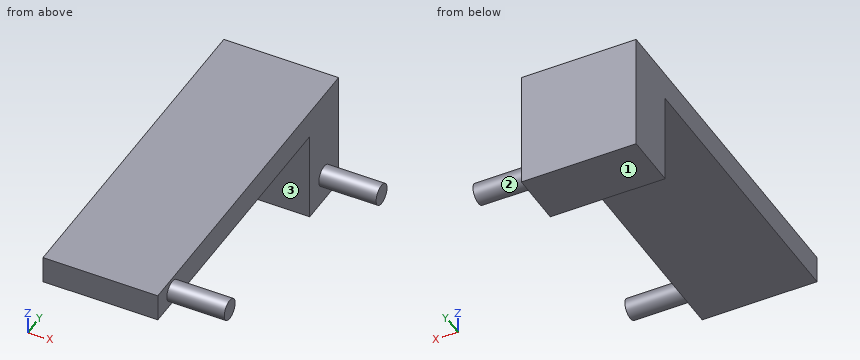
```python
from build123d import *

# Parameters (mm, degrees)
F0_W     = 50
F0_H     = 150
F1_DEPTH = 12
F2_W     = 24
F2_H     = 40
F3_DEPTH = 50
F4_R     = 4.5
F5_DEPTH = 25


with BuildPart() as f1:
    # F0 (on Top) → F1 (new body)
    with BuildSketch(Plane.XY):
        Rectangle(F0_W, F0_H)
    extrude(amount=F1_DEPTH)

    # F2 (on face) → F3 (join)
    with BuildSketch(Plane.YZ.offset(25)):
        with Locations((63, -20)):
            Rectangle(F2_W, F2_H)
    extrude(amount=-F3_DEPTH)

    # F4 (on face) → F5 (join)
    with BuildSketch(Plane.YZ.offset(25)):
        with Locations((-63, 6)):
            Circle(F4_R)
        with Locations((63, -28)):
            Circle(F4_R)
    extrude(amount=F5_DEPTH)


solid = f1.part
```
Check sheet for the modelled part. Datum: model origin and axes. Units: mm. Face numbers are marked on the shaded views. A direction names the side the tool comes from. Give positions to 0.01 mm unless a question says otherwise; leave off trailing zeros. Write each loop counter-clockwise with the first axis right and the second up, starting at its lowest first coordinate (ties: lowest second). Pieces come first, ordered by that corner, then holes. Notation, with made-up numbers: (55.25, -3.75) - (76.25, -3.75) arc R20 ccw to (76.25, 29.25) - close; hole circle Ø6 at (76, 47.5). An arc over 180 degrees is marked (long way). Answer as a JSON object with one key per item and string values. Group by question number.
1) Depth check by flat-ended pin: P1, Ø12, axis at x = -9, z = -25, coming from the -Y side; P2, Ø15, axis at x = 7, y = -32, coming from the -Z side. Enter the tip coordinate at first touch or a pass-through.
2) Sectioned sample at B-B (z = 6). Record the cut outline in (x, y).
3) Thickness scan on probe 1 along Z at (x, y) = (-16, 46); probe 2 along X at (y, z) = (69, -19); probe 3 along Y at (x, z) = (-7, -36). Record the ranges inside material, lowest first. Write a range as from..to.
4) Sectioned sample at A-A (y = 63). Record the cut outline in (x, z), then the cut area to 4 significant figures.
5) Sectioned sample at D-D (y = -16). Record the cut outline in (x, z), then the cut area to 3 significant figures.
6) Access from +Z, -Z, +X, -X, +Y, -Y to the whole of each face (thin tool, end or side, straight path). Record for the marked faces 1, 2 and 3.
7) Sectioned sample at C-C (x = -4.5). Record the cut outline in (y, z).
Geometry results:
{
 "1": {"P1": "stops at y = 51", "P2": "stops at z = 0"},
 "2": {"outline": "(-25, -75) - (25, -75) - (25, -67.5) - (50, -67.5) - (50, -58.5) - (25, -58.5) - (25, 75) - (-25, 75) - close"},
 "3": {"probe 1": "z = 0..12", "probe 2": "x = -25..25", "probe 3": "y = 51..75"},
 "4": {"outline": "(-25, -40) - (25, -40) - (25, -32.5) - (50, -32.5) - (50, -23.5) - (25, -23.5) - (25, 12) - (-25, 12) - close", "area": "2,825 mm^2"},
 "5": {"outline": "(-25, 0) - (25, 0) - (25, 12) - (-25, 12) - close", "area": "600 mm^2"},
 "6": {"face 1": "-Z, +X, -X, +Y, -Y", "face 2": "+X", "face 3": "-Z, +X, -X, -Y"},
 "7": {"outline": "(-75, 0) - (51, 0) - (51, -40) - (75, -40) - (75, 12) - (-75, 12) - close"}
}
